Build history of the part. All positions in model axes, mm. A direction names the side the tool comes from. Round coordinates to 2 decimals unless told otherwise and drop trailing zeros. Order: outer loops, then holes, each group sorted by start corner. A loop starts at its lowest first (then second) coordinate and runs counter-clockwise, first axis right, second up. Notation, with made-up numbers: (22, 41) -> (79, 41) arc R25 cw to (79, 66) -> close; hole circle Ø8 at (-22.5, 47.25). An arc over 180 degrees is marked (long way). Use a Markdown table: item, result. Add a question column.
Item 1: Two-plate mould, pull along Y, no slides. Class faces 1 (the face through (5.27, 2.96, 1.87)), 2 (the face through (3.11, 1.84, 2.99)), 3 (the face through (3, 2, 0)): released by +Y, released by -Y, zero draft, split by the parting line, or undercut.
Item 2: Slice it at C-C, the plane x = 6.5. Give the cut face in (y, z).
Item 3: Probe L1, parallel to Y at x = 2, z = 3.6; L2, parallel to X at y = 1.2, z = 2.6; L3, parallel to Y at x = 2.5, z = 3.25. List the from-to ranges inside material, lowest first.
Item 4: Slice it at B-B, the plane y = 3.15. Give the cut face in (x, z), plus the area to 3 significant figures.
Item 5: Slice it at A-A, the plane z = 2.8. Give the cut face in (x, y), plus the area to 3 significant figures.
Item 6: Slice it at D-D, the plane z = 1.85. Give the cut face in (x, y), plus the area to 3 significant figures.
Item 7: 3-axis set-ups, long thin cutter, end or side, ignore diameter. For faces 4 (the face through (3.303, 1.961, 2.986)), 5 (the face through (2, 1, 4)): which of +Z, -Z, +X, -X, +Y, -Y reach the whole face in a straight line?
from build123d import *

# Parameters (mm, degrees)
BOSS_EXTRUDE1_DEPTH  = 4
CUT_SWEEP1_START     = 3.150069302
CUT_SWEEP1_OUTLINE_W = 8
CUT_SWEEP1_OUTLINE_H = 2
CUT_SWEEP1_DEPTH     = 0.2000044
CHAMFER1_SIZE        = 0.2


# Read off the part's stored shape, not the designer's step: Cut-Sweep1
with BuildPart() as part:
    # Sketch1 → Boss-Extrude1 (new body)
    with BuildSketch(Plane.XY):
        Polygon((0, 0), (10.4, 0), (0, 6), align=None)
    extrude(amount=BOSS_EXTRUDE1_DEPTH)

    # Cut-Sweep1 outline → Cut-Sweep1 (cut)
    with BuildSketch(Plane(origin=(0, 0, 0), x_dir=(0.866019052628739, -0.5000110003630132, 0), z_dir=(0.5000110003630132, 0.8660190526287392, 0)).offset(CUT_SWEEP1_START)):
        with Locations((2, -3)):
            Rectangle(CUT_SWEEP1_OUTLINE_W, CUT_SWEEP1_OUTLINE_H)
    extrude(amount=CUT_SWEEP1_DEPTH, mode=Mode.SUBTRACT)

    # Chamfer1
    chamfer1_edges = [part.edges().sort_by_distance(p)[0] for p in [
        (5.2, 3, 4),
    ]]
    chamfer(chamfer1_edges, length=CHAMFER1_SIZE)


solid = part.part
Check sheet entries:
| question | item | result |
|---|---|---|
| 1 | face 1 | released by +Y |
| 1 | face 2 | undercut |
| 1 | face 3 | zero draft |
| 2 | outline | (0, 0) -> (2.25, 0) -> (2.25, 3.8) -> (2.02, 4) -> (0.12, 4) -> (0.12, 2) -> (0, 2) -> close |
| 3 | L1 | 0 to 2.48, 2.71 to 4.85 |
| 3 | L2 | 0 to 4.22, 4.62 to 8.32 |
| 3 | L3 | 0 to 2.19, 2.42 to 4.56 |
| 4 | outline | (0, 0) -> (4.94, 0) -> (4.94, 3.8) -> (4.54, 4) -> (1.24, 4) -> (1.24, 2) -> (0.84, 2) -> (0.84, 4) -> (0, 4) -> close |
| 4 | area | 18.9 mm2 |
| 5 | outline | (0, 0) -> (6.3, 0) -> (0, 3.64) -> close; (0, 3.87) -> (6.7, 0) -> (10.4, 0) -> (0, 6) -> close |
| 5 | area | 29.7 mm2 |
| 6 | outline | (0, 0) -> (10.4, 0) -> (0, 6) -> close |
| 6 | area | 31.2 mm2 |
| 7 | face 4 | +Z |
| 7 | face 5 | +Z, +X, -X, +Y, -Y |
